Source: CAD feature listing. Evaluate the final solid. Frame: model axes, mm. Give positions to 0.01 mm unless a question says otherwise; leave off trailing zeros. Write each loop counter-clockwise with the first axis right and the second up, starting at its lowest first coordinate (ties: lowest second). Pieces come first, ordered by that corner, then holes. Notation, with made-up numbers: (24.5, 6) -> (75.5, 6) arc R15 ccw to (75.5, 19) -> close; hole circle Ø5 at (61.25, -28.5). An arc over 180 degrees is marked (long way). Use a Markdown table: item, result. Add a question column.
```python
from build123d import *

# Parameters (mm, degrees)
F0_W     = 127
F0_H     = 50.8
F2_W     = 19.05
F2_H     = 63.5
F3_DEPTH = 50.801
F4_R     = 12.7
F5_DEPTH = 50.801
F6_R     = 5.08


with BuildPart() as f1:
    # F0 (on Front) → F1 (revolve)
    with BuildSketch(Plane.XZ):
        with Locations((63.5, 25.4)):
            Rectangle(F0_W, F0_H)
    revolve(axis=Axis((0, 0, 25.4), (0, 0, 1)))

    # F2 (on face) → F3 (cut, through all)
    with BuildSketch(Plane.XY.offset(50.8)):
        with Locations((0, 63.5)):
            Rectangle(F2_W, F2_H)
        with Locations((0, -63.5)):
            Rectangle(F2_W, F2_H)
    extrude(amount=-F3_DEPTH, mode=Mode.SUBTRACT)

    # F4 (on face) → F5 (cut, through all)
    with BuildSketch(Plane.XY.offset(50.8)):
        Circle(F4_R)
    extrude(amount=-F5_DEPTH, mode=Mode.SUBTRACT)

    # F6
    f6_edges = [f1.edges().sort_by_distance(p)[0] for p in [
        (-127, 0, 50.8),
        (9.525, -63.5, 50.8),
        (0, -95.25, 50.8),
        (-9.525, -63.5, 50.8),
        (0, -31.75, 50.8),
        (-12.7, 0, 50.8),
        (0, 95.25, 50.8),
        (9.525, 63.5, 50.8),
        (-9.525, 63.5, 50.8),
        (0, 31.75, 50.8),
        (-127, 0, 0),
        (9.525, -63.5, 0),
        (0, -95.25, 0),
        (-9.525, -63.5, 0),
        (0, -31.75, 0),
        (-12.7, 0, 0),
        (0, 31.75, 0),
        (9.525, 63.5, 0),
        (-9.525, 63.5, 0),
        (0, 95.25, 0),
    ]]
    fillet(f6_edges, radius=F6_R)


solid = f1.part
```
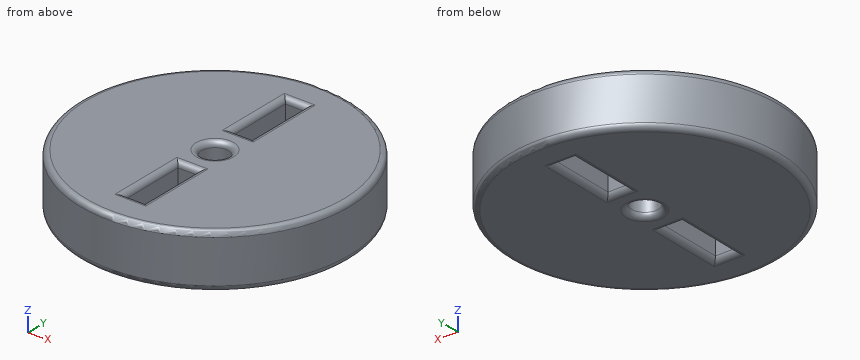
(1) Cut plane A-A on y = 0. Return the cut outline in (x, z).
(2) Cut plane B-B on x = 0. Count the separate pieces of the cut face and the enclosed holes in it, then the cut area to 3 significant figures.
(3) Material intervals for L1, parallel to Y at x = 0, z = 24; L2, parallel to X at y = -6, z = 7.5; L3, parallel to X at y = 63, z = 9.5 (3 decimals), sorted ascending.
(4) Cut plane C-C on z = 40. Return the cut outline in (x, y) (3 decimals).
(5) First-contact query: pin 1 Ø1 at (x, z) = (-89.5, 43) entering from +Y; pin 2 Ø20.5 at (y, z) = (60.5, 19) entering from +X; pin 3 Ø2 at (y, z) = (11, 18) entering from +X; pin 4 Ø6 at (y, z) = (-1.5, 29) entering from +X. Flat tips, straight axial feed; report the tip coordinate or a pass-through.
Output:
| question | item | result |
|---|---|---|
| 1 | outline | (-127, 5.08) arc R5.08 ccw to (-121.92, 0) -> (-17.78, 0) arc R5.08 ccw to (-12.7, 5.08) -> (-12.7, 45.72) arc R5.08 ccw to (-17.78, 50.8) -> (-121.92, 50.8) arc R5.08 ccw to (-127, 45.72) -> close; (12.7, 5.08) arc R5.08 ccw to (17.78, 0) -> (121.92, 0) arc R5.08 ccw to (127, 5.08) -> (127, 45.72) arc R5.08 ccw to (121.92, 50.8) -> (17.78, 50.8) arc R5.08 ccw to (12.7, 45.72) -> close |
| 2 | separate pieces | 4 |
| 2 | enclosed holes | 0 |
| 2 | area | 5,070 mm^2 |
| 3 | L1 | -127 to -95.25, -31.75 to -12.7, 12.7 to 31.75, 95.25 to 127 |
| 3 | L2 | -126.86 to -11.19, 11.19 to 126.86 |
| 3 | L3 | -110.272 to -9.525, 9.525 to 110.272 |
| 4 | outline | circle Ø254 at (0, 0); hole circle Ø25.4 at (0, 0); hole (-9.525, -95.25) -> (9.525, -95.25) -> (9.525, -31.75) -> (-9.525, -31.75) -> close; hole (-9.525, 31.75) -> (9.525, 31.75) -> (9.525, 95.25) -> (-9.525, 95.25) -> close |
| 5 | pin 1 | y = 90.6 |
| 5 | pin 2 | x = 116.64 |
| 5 | pin 3 | x = 126.61 |
| 5 | pin 4 | x = 127 |
